Here's how the part is built. I have some questions about the finished solid (model axes, mm). A direction names the side the tool comes from. Give positions to 0.01 mm unless a question says otherwise; leave off trailing zeros. Order: outer loops, then holes, each group sorted by start corner. A loop starts at its lowest first (then second) coordinate and runs counter-clockwise, first axis right, second up. Notation, with made-up numbers: (82.5, 40.25) - (108.5, 40.25) arc R7 ccw to (108.5, 50.25) - close; hole circle Ø9 at (-17.75, -12.75). An arc over 180 degrees is marked (long way). One line per question, with ' | ' between items.
from build123d import *

# Parameters (mm, degrees)
SKETCH2_R           = 4
SKETCH2_R_2         = 2
BOSS_EXTRUDE1_DEPTH = 7


with BuildPart() as part:
    # Sketch2 → Boss-Extrude1 (new body, symmetric)
    with BuildSketch(Plane.XY):
        with BuildLine():
            Line((-6.131872753, 29.88679476), (5.868127247, 29.88679476))
            Line((5.868127247, 29.88679476), (7.594498309, 29.88679476))
            Line((7.594498309, 29.88679476), (8.387086053, 29.88679476))
            Line((8.387086053, 29.88679476), (8.387086053, 29.094207016))
            Line((8.387086053, 29.094207016), (17.251890726, 23.08634601))
            Line((17.251890726, 23.08634601), (17.251890726, 20.138485624))
            Line((17.251890726, 20.138485624), (17.251890726, 4.758566897))
            Line((17.251890726, 4.758566897), (17.251890726, 3.572124473))
            Line((17.251890726, 3.572124473), (12.798407994, 3.572124473))
            Line((12.798407994, 3.572124473), (10.603625269, 1.11753322))
            Line((10.603625269, 1.11753322), (10.603625269, -1.34605728))
            Line((10.603625269, -1.34605728), (10.581729624, -12.61320524))
            Line((10.581729624, -12.61320524), (10.581729624, -21.11320524))
            Line((10.581729624, -21.11320524), (-2.916105285, -21.11320524))
            Line((-2.916105285, -21.11320524), (-2.916105285, -12.61320524))
            Line((-2.916105285, -12.61320524), (-2.916105285, -2.61320524))
            ThreePointArc((-2.916105285, -2.61320524), (-3.030865934, -1.996216384), (-3.359797705, -1.461754837))
            Line((-3.359797705, -1.461754837), (-3.359797705, 2.88679476))
            Line((-3.359797705, 2.88679476), (-12.040045413, 2.88679476))
            ThreePointArc((-12.040045413, 2.88679476), (-13.161439875, 4.684724171), (-15.160732898, 5.38679476))
            Line((-15.160732898, 5.38679476), (-14.332399999, 5.38679476))
            ThreePointArc((-14.332399999, 5.38679476), (-15.333457628, 5.801446406), (-15.748109274, 6.802504035))
            Line((-15.748109274, 6.802504035), (-15.748109274, 20.089109399))
            Line((-15.748109274, 20.089109399), (-15.748109274, 21.453992916))
            Line((-15.748109274, 21.453992916), (-13.659474375, 21.453992916))
            ThreePointArc((-13.659474375, 21.453992916), (-12.819577694, 21.664599805), (-12.178425993, 22.246584507))
            Line((-12.178425993, 22.246584507), (-7.612913947, 29.094207016))
            ThreePointArc((-7.612913947, 29.094207016), (-6.971765358, 29.676188893), (-6.131872753, 29.88679476))
        make_face()
        with Locations((-6.213784577, 13.445806717)):
            Circle(SKETCH2_R, mode=Mode.SUBTRACT)
        with Locations((11.786215423, 13.445806717)):
            Circle(SKETCH2_R_2, mode=Mode.SUBTRACT)
        with Locations((-6.131872753, 25.90633221)):
            Circle(SKETCH2_R_2, mode=Mode.SUBTRACT)
        with Locations((5.868127247, 25.90633221)):
            Circle(SKETCH2_R_2, mode=Mode.SUBTRACT)
    extrude(amount=BOSS_EXTRUDE1_DEPTH, both=True)


solid = part.part
1) I want a section at B-B (z = 2.5). List the corners of the cut face in (x, y) for me.
Model answer:
outline: (-15.75, 6.8) arc R1.42 ccw to (-14.33, 5.39) - (-15.16, 5.39) arc R3.2 cw to (-12.04, 2.89) - (-3.36, 2.89) - (-3.36, -1.46) arc R1.72 cw to (-2.92, -2.61) - (-2.92, -21.11) - (10.58, -21.11) - (10.58, -12.61) - (10.6, -1.35) - (10.6, 1.12) - (12.8, 3.57) - (17.25, 3.57) - (17.25, 23.09) - (8.39, 29.09) - (8.39, 29.89) - (-6.13, 29.89) arc R1.78 ccw to (-7.61, 29.09) - (-12.18, 22.25) arc R1.78 cw to (-13.66, 21.45) - (-15.75, 21.45) - close; hole circle Ø8 at (-6.21, 13.45); hole circle Ø4 at (-6.13, 25.91); hole circle Ø4 at (5.87, 25.91); hole circle Ø4 at (11.79, 13.45)
2) On a 3-axis mill with a long thin cutter (end or side, diameter ignored), from which of +Z, -Z, +X, -X, +Y, -Y can I reach the whole of each face in a straight line? I mean faces 1 (the face through (-15, 21.454, 0)), 2 (the face through (15, 3.572, 0)), 3 (the face through (-2.916, -12, 0)). Say none if no direction works.
Model answer:
face 1: +Z, -Z, -X, +Y | face 2: +Z, -Z, +X, -Y | face 3: +Z, -Z, -X, -Y
3) I'm going to push flat-ended pins straight in: P1, Ø1, axis at x = -14.5, z = 0, coming from the +Y side; P2, Ø1.5, axis at x = -7.5, z = 3.5, coming from the +Y side; P3, Ø3, axis at x = -6.13, y = 25.91, coming from the +Z side; P4, Ø5, axis at x = 14.5, z = -0.5, coming from the -Y side. Where does each tip first touch, or does it pass through?
Model answer:
P1: stops at y = 21.45 | P2: stops at y = 29.78 | P3: passes through | P4: stops at y = 2.68
4) I want a section at D-D (y = -0.5). List the corners of the cut face in (x, z) for me.
Model answer:
outline: (-3.36, -7) - (10.6, -7) - (10.6, 7) - (-3.36, 7) - close
5) I want a section at C-C (x = -7). List the corners of the cut face in (y, z) for me.
Model answer:
outline: (2.89, -7) - (9.52, -7) - (9.52, 7) - (2.89, 7) - close; (17.37, -7) - (24.1, -7) - (24.1, 7) - (17.37, 7) - close; (27.71, -7) - (29.66, -7) - (29.66, 7) - (27.71, 7) - close
6) I want a section at A-A (y = 25). List the corners of the cut face in (x, z) for me.
Model answer:
outline: (-10.34, -7) - (-7.91, -7) - (-7.91, 7) - (-10.34, 7) - close; (-4.35, -7) - (4.09, -7) - (4.09, 7) - (-4.35, 7) - close; (7.65, -7) - (14.43, -7) - (14.43, 7) - (7.65, 7) - close
7) Thinking about a two-plate mould opening in X: for faces 4 (the face through (1, 29.887, 0)), 5 (the face through (10.604, 0, 0)), 6 (the face through (10.2, 12.23, -0.1)), which applies, +X half, -X half, draft (parallel to the pull), parting line (faces both ways), or undercut?
Model answer:
face 4: draft | face 5: +X half | face 6: undercut
8) Please list where these lines run through material, in increasing order: L1, parallel to Y at x = -7, z = -2.25; L2, parallel to X at y = -11.5, z = 3.25; L3, parallel to Y at x = 6.5, z = -6.5.
Model answer:
L1: y = 2.89 to 9.52, 17.37 to 24.1, 27.71 to 29.66 | L2: x = -2.92 to 10.58 | L3: y = -21.11 to 24.01, 27.8 to 29.89
